Check sheet for the drawn part. Datum: minimum x, y, z corner. Units: mm. Give positions to 0.01 mm unless a question says otherwise; leave off trailing zeros. Loops run counter-clockwise (first coordinate to the right, second up) from the corner with the lowest first, then second, coordinate; pieces in that order, holes last. Notation, with made-up numbers: (-7, 49.25) - (29, 49.25) arc R37 ccw to (29, 88.25) - close; hole circle Ø5 at (54, -27). An arc over 180 degrees is marked (long way). Use a Markdown table: item, result. Add a question column.
1. Material ranges on L1, parallel to X at y = 10.25, z = 8.5 (1 decimal); L2, parallel to X at y = 13.25, z = 18 (1 decimal), recorded low to high.
2. Draft check along Y on the marked faces 1 and 2. Enter one of: pulls with the +Y half, pulls with the -Y half, needs draft (parallel to the pull), parting line crosses it, or undercut.
3. Cross-section at A-A on z = 11. Enter the section's corners in (x, y) (1 decimal).
4. Depth check by flat-ended pin: P1, Ø1.5, axis at x = 15, z = 35.5, coming from the +Y side; P2, Ø3, axis at y = 16, z = 50.5, coming from the +X side; P3, Ø1.5, axis at y = 7, z = 40.5, coming from the -X side. Enter the tip coordinate at first touch or a pass-through.
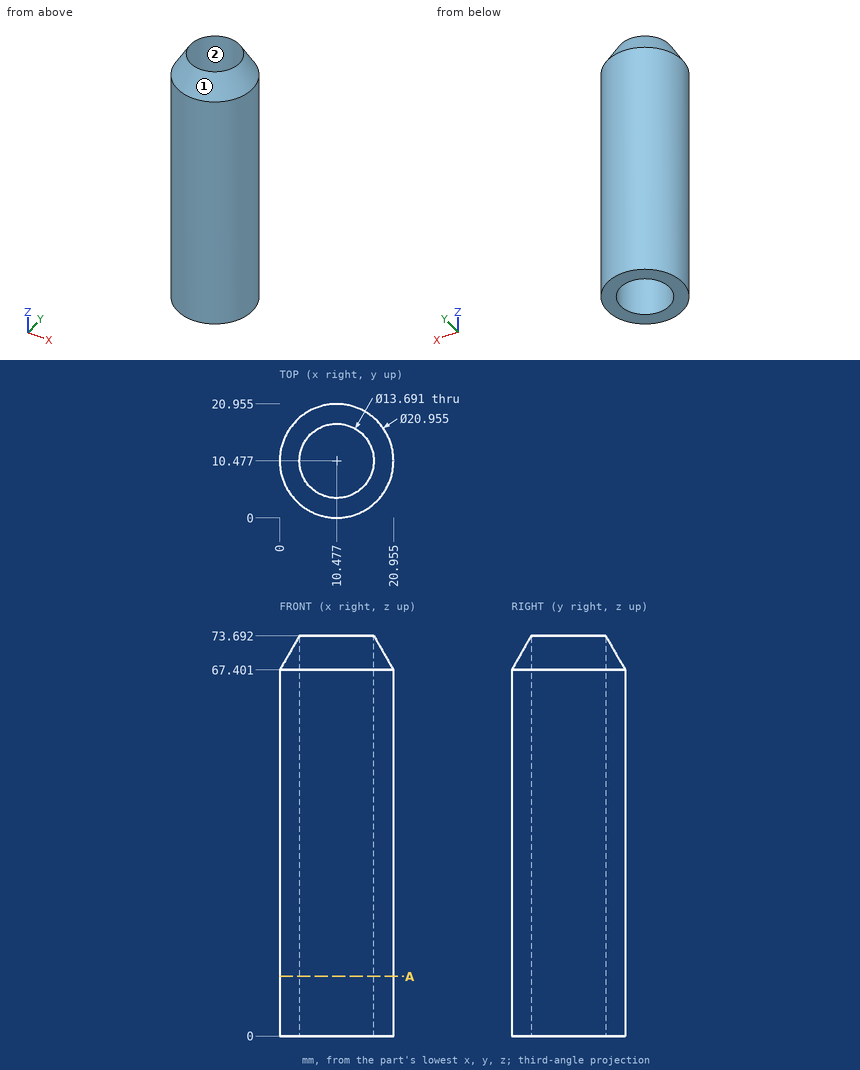
Values found:
| question | item | result |
|---|---|---|
| 1 | L1 | x = 0 to 3.6, 17.3 to 21 |
| 1 | L2 | x = 0.4 to 4.2, 16.7 to 20.6 |
| 2 | face 1 | parting line crosses it |
| 2 | face 2 | undercut |
| 3 | outline | circle Ø21 at (10.5, 10.5); hole circle Ø13.7 at (10.5, 10.5) |
| 4 | P1 | stops at y = 20.25 |
| 4 | P2 | stops at x = 20.15 |
| 4 | P3 | stops at x = 0.36 |
